CAD build for the part. Positions are in the model's coordinates, mm. A direction names the side the tool comes from. Round coordinates to 2 decimals unless told otherwise and drop trailing zeros. Write each loop counter-clockwise with the first axis right and the second up, starting at its lowest first coordinate (ties: lowest second). Pieces come first, ordered by that corner, then holes. Notation, with made-up numbers: (-21.5, 27.25) - (37.5, 27.25) arc R28 cw to (37.5, 64.25) - close; hole circle Ø7 at (44, 43.25). An arc over 180 degrees is marked (long way). Use one line per item in the form item = value. Start each with the question number.
Item 1: Band-saw the part on C-C, the plane z = -19.5. List the corners of the cut face in (x, y), and give its area (3 significant figures).
Item 2: Pin check, flat tips, straight feed: pin 1 (2 mm diameter, centred on x = 18.5, y = 2.5, fed in from -Z); pin 2 (1 mm diameter, centred on y = 2, z = 15, fed in from -X); pin 3 (1.4 mm diameter, centred on x = 21, y = 2.5, fed in from +Z). Stop position of each tip, or through.
Item 3: Band-saw the part on D-D, the plane y = 1.7. Give the number of separate pieces and of enclosed holes in the cut face, and give its area (3 significant figures).
Item 4: Pull direction Z, two halves, no side cores. Call faces 3 (the cylindrical face through (-23.48, 2.96, -0.99)), 4 (the flat face through (-10.2, 0, -0.3)), 5 (the cylindrical face through (11.11, 2.96, 15.4)): +Z half, -Z half, draft (parallel to the pull), parting line (faces both ways), or undercut.
Item 5: Drill centre lines: L1, parallel to X at y = 4.3, z = 0 (3 decimals); L2, parallel to Z at x = 17.5, y = 2.5; L3, parallel to X at y = 1.5, z = -18. Where is each one in solid material? Low to high.
Item 6: Band-saw the part on B-B, the plane x = -3. List the corners of the cut face in (y, z), and give its area (3 significant figures).
Item 7: Tool access for faces 1 (the flat face through (20, 3, -2)), 2 (the cylindrical face through (-16.8, 3, -11.8)): list every direction of +Z, -Z, +X, -X, +Y, -Y with a clear straight run to the whole face (end or side of a thin tool).
Item 8: Band-saw the part on A-A, the plane z = 0. List the corners of the cut face in (x, y) (3 decimals), and give its area (3 significant figures).
from build123d import *

# Parameters (mm, degrees)
SKETCH_1_R          = 23.5
SKETCH_1_R_2        = 10
SKETCH_1_R_3        = 2.05
SKETCH_1_R_4        = 2.015
EXTRUDE_1_DEPTH     = 6
SKETCH_2_W          = 12.240085516
SKETCH_2_H          = 4
CUT_EXTRUDE_1_DEPTH = 10
FILLET_1_R          = 1


with BuildPart() as part:
    # 草图1 → 凸台-拉伸1 (new body)
    with BuildSketch(Plane(origin=(0, 0, 0), x_dir=(1, 0, 0), z_dir=(0, 1, 0))):
        with Locations(Location((0, 0, 0), (0, 0, 270))):
            Circle(SKETCH_1_R)
        with Locations(Location((0, 0, 0), (0, 0, 270))):
            Circle(SKETCH_1_R_2, mode=Mode.SUBTRACT)
        with Locations(Location((0, 19.5, 0), (0, 0, 270))):
            Circle(SKETCH_1_R_3, mode=Mode.SUBTRACT)
        with Locations(Location((16.887495374, 9.75, 0), (0, 0, 270))):
            Circle(SKETCH_1_R_3, mode=Mode.SUBTRACT)
        with Locations(Location((16.887495374, -9.75, 0), (0, 0, 270))):
            Circle(SKETCH_1_R_3, mode=Mode.SUBTRACT)
        with Locations(Location((0, -19.5, 0), (0, 0, 270))):
            Circle(SKETCH_1_R_3, mode=Mode.SUBTRACT)
        with Locations(Location((-16.887495374, -9.75, 0), (0, 0, 270))):
            Circle(SKETCH_1_R_3, mode=Mode.SUBTRACT)
        with Locations(Location((-16.887495374, 9.75, 0), (0, 0, 270))):
            Circle(SKETCH_1_R_3, mode=Mode.SUBTRACT)
        with Locations(Location((-19.5, 0, 0), (0, 0, 270))):
            Circle(SKETCH_1_R_4, mode=Mode.SUBTRACT)
        with Locations(Location((9.75, 16.887495374, 0), (0, 0, 270))):
            Circle(SKETCH_1_R_4, mode=Mode.SUBTRACT)
        with Locations(Location((9.75, -16.887495374, 0), (0, 0, 270))):
            Circle(SKETCH_1_R_4, mode=Mode.SUBTRACT)
    extrude(amount=EXTRUDE_1_DEPTH)

    # 草图2 → 切除-拉伸1 (cut)
    with BuildSketch(Plane(origin=(0, 6, 0), x_dir=(1, 0, 0), z_dir=(0, 1, 0))):
        with Locations((22.620042758, 0)):
            Rectangle(SKETCH_2_W, SKETCH_2_H)
    extrude(amount=-CUT_EXTRUDE_1_DEPTH, mode=Mode.SUBTRACT)

    # 圆角1
    fillet_1_edges = [part.edges().sort_by_distance(p)[0] for p in [
        (23.414738948, 3, 2),
        (23.414738948, 3, -2),
        (16.5, 3, 2),
        (16.5, 3, -2),
    ]]
    fillet(fillet_1_edges, radius=FILLET_1_R)


solid = part.part
Determined:
q1.outline = (-13.11, 0) - (-2.05, 0) - (-2.05, 6) - (-13.11, 6) - close; (2.05, 0) - (13.11, 0) - (13.11, 6) - (2.05, 6) - close
q1.area = 133 mm²
q2.pin_1 = -15.68
q2.pin_2 = -18.49
q2.pin_3 = 11.84
q3.separate_pieces = 1
q3.enclosed_holes = 10
q3.area = 1,280 mm²
q4.face_3 = parting line
q4.face_4 = draft
q4.face_5 = undercut
q5.L1 = -23.5 to -21.515, -17.485 to -10, 10 to 16.5
q5.L2 = -15.68 to -11.71, -7.79 to -2, 2 to 7.79, 11.71 to 15.68
q5.L3 = -15.11 to -1.4, 1.4 to 8.07, 11.43 to 15.11
q6.outline = (0, -23.31) - (6, -23.31) - (6, -9.54) - (0, -9.54) - close; (0, 9.54) - (6, 9.54) - (6, 23.31) - (0, 23.31) - close
q6.area = 165 mm²
q7.face_1 = +X, +Y, -Y
q7.face_2 = +Y, -Y
q8.outline = (-23.5, 0) - (-21.515, 0) - (-21.515, 6) - (-23.5, 6) - close; (-17.485, 0) - (-10, 0) - (-10, 6) - (-17.485, 6) - close; (10, 0) - (16.5, 0) - (16.5, 6) - (10, 6) - close
q8.area = 95.8 mm²
